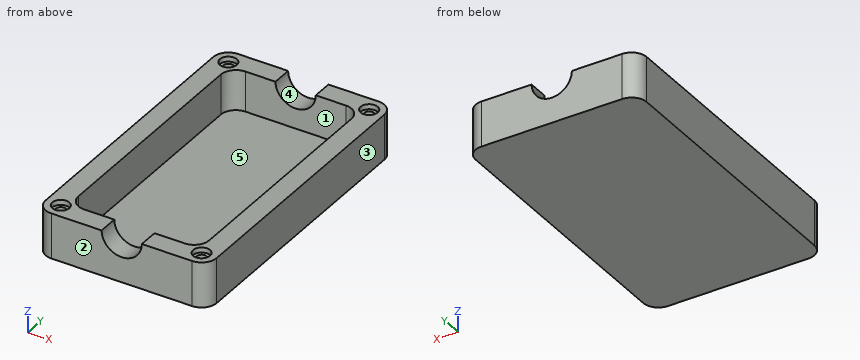
```python
from build123d import *

# Parameters (mm, degrees)
SKETCH008_W                   = 34
SKETCH008_H                   = 59
PAD002_DEPTH                  = 9
SKETCH009_W                   = 26
SKETCH009_H                   = 51
POCKET005_DEPTH               = 8
FILLET003_R                   = 3
SKETCH010_R                   = 1
POCKET006_DEPTH               = 4
SKETCH010_MIRRORED004_2_R     = 1
POCKET006_MIRRORED004_2_DEPTH = 4
SKETCH011_R                   = 1.7
POCKET007_DEPTH               = 1
SKETCH011_MIRRORED006_2_R     = 1.7
POCKET007_MIRRORED006_2_DEPTH = 1
SKETCH016_R                   = 4
POCKET011_DEPTH               = 59.001


with BuildPart() as part:
    # Sketch008 → Pad002 (new body)
    with BuildSketch(Plane.XY):
        Rectangle(SKETCH008_W, SKETCH008_H)
    extrude(amount=PAD002_DEPTH)

    # Sketch009 (on Face6 of Pad002) → Pocket005 (cut)
    with BuildSketch(Plane.XY.offset(9)):
        Rectangle(SKETCH009_W, SKETCH009_H)
    extrude(amount=-POCKET005_DEPTH, mode=Mode.SUBTRACT)

    # Fillet003
    fillet003_edges = [part.edges().sort_by_distance(p)[0] for p in [
        (-13, 25.5, 5),
        (-17, 29.5, 4.5),
        (17, 29.5, 4.5),
        (13, 25.5, 5),
        (17, -29.5, 4.5),
        (13, -25.5, 5),
        (-13, -25.5, 5),
        (-17, -29.5, 4.5),
    ]]
    fillet(fillet003_edges, radius=FILLET003_R)

    # Sketch010 (on Face5 of Fillet003) → Pocket006 (cut)
    with BuildSketch(Plane.XY.offset(9)):
        with Locations((-14, 26.5)):
            Circle(SKETCH010_R)
    pocket006 = extrude(amount=-POCKET006_DEPTH, mode=Mode.SUBTRACT)

    # Sketch010 Mirrored004 2 → Pocket006 Mirrored004 2 (cut)
    with BuildSketch(Plane(origin=(0, 0, 9), x_dir=(-1, 0, 0), z_dir=(0, 0, -1))):
        with Locations((-14, 26.5)):
            Circle(SKETCH010_MIRRORED004_2_R)
    pocket006_mirrored004_2 = extrude(amount=POCKET006_MIRRORED004_2_DEPTH, mode=Mode.SUBTRACT)

    # Mirrored005: Pocket006, Pocket006 Mirrored004 2 across Sketch010 H_Axis
    add(pocket006.mirror(Plane(origin=(0, 0, 9), x_dir=(0, 0, 1), z_dir=(0, 1, 0))), mode=Mode.SUBTRACT)
    add(pocket006_mirrored004_2.mirror(Plane(origin=(0, 0, 9), x_dir=(0, 0, 1), z_dir=(0, 1, 0))), mode=Mode.SUBTRACT)

    # Sketch011 (on Face5 of MultiTransform002) → Pocket007 (cut)
    with BuildSketch(Plane.XY.offset(9)):
        with Locations((-14, 26.5)):
            Circle(SKETCH011_R)
    pocket007 = extrude(amount=-POCKET007_DEPTH, mode=Mode.SUBTRACT)

    # Sketch011 Mirrored006 2 → Pocket007 Mirrored006 2 (cut)
    with BuildSketch(Plane(origin=(0, 0, 9), x_dir=(-1, 0, 0), z_dir=(0, 0, -1))):
        with Locations((-14, 26.5)):
            Circle(SKETCH011_MIRRORED006_2_R)
    pocket007_mirrored006_2 = extrude(amount=POCKET007_MIRRORED006_2_DEPTH, mode=Mode.SUBTRACT)

    # Mirrored007: Pocket007, Pocket007 Mirrored006 2 across Sketch011 H_Axis
    add(pocket007.mirror(Plane(origin=(0, 0, 9), x_dir=(0, 0, 1), z_dir=(0, 1, 0))), mode=Mode.SUBTRACT)
    add(pocket007_mirrored006_2.mirror(Plane(origin=(0, 0, 9), x_dir=(0, 0, 1), z_dir=(0, 1, 0))), mode=Mode.SUBTRACT)

    # Sketch016 (on Face10 of MultiTransform003) → Pocket011 (cut, through all)
    with BuildSketch(Plane.XZ.offset(29.5)):
        with Locations((0, 9)):
            Circle(SKETCH016_R)
    extrude(amount=-POCKET011_DEPTH, mode=Mode.SUBTRACT)


solid = part.part
```
Read the model definition and answer for the solid it produces. Units are mm, in the model's axes. Face numbers are marked on the shaded views. A direction names the side the tool comes from. Give positions to 0.01 mm unless a question says otherwise; leave off trailing zeros. Loops run counter-clockwise (first coordinate to the right, second up) from the corner with the lowest first, then second, coordinate; pieces in that order, holes last.
Item 1: Find the intervals of material crossed by line 1 along Y through (x, z) = (-14, 6.25); line 2 along X through (y, z) = (-12.5, 8.5); line 3 along Z through (x, y) = (10.5, -0.5), in increasing order.
Item 2: The part is cut by section A-A (z = 6.75). Write down the section's boundary in (x, y), and give its area (3 significant figures).
Item 3: For the marked faces 4 and 5, determine the directions among +Z, -Z, +X, -X, +Y, -Y from which every point of the face is accessible in a straight line to the end or side of a thin tool.
Item 4: The part is cut by section B-B (y = -2). Write down the section's boundary in (x, z).
Item 5: The mould has two halves that part along Y. Classify the marked faces 1, 2 and 3: released by +Y, released by -Y, zero draft, split by the parting line, or undercut.
Item 6: The part is cut by section C-C (z = 3.5). Write down the section's boundary in (x, y).
Item 7: The part is cut by section D-D (x = -1.5). Write down the section's boundary in (y, z).
Item 8: Each of these flat-tipped pins is pushed along its axis until it touches: pin 1 Ø1 at (x, y) = (-14.5, -26) entering from +Z; pin 2 Ø6 at (x, y) = (8, -8) entering from +Z; pin 3 Ø1.6 at (x, y) = (14, -26.5) entering from +Z. Where does it stop, or does it pass through?
Taken from the geometry:
1. line 1: y = -29.5 to -27.5, -25.5 to 25.5, 27.5 to 29.5
1. line 2: x = -17 to -13, 13 to 17
1. line 3: z = 0 to 1
2. outline: (-17, -26.5) arc R3 ccw to (-14, -29.5) - (-3.31, -29.5) - (-3.31, -25.5) - (-10, -25.5) arc R3 cw to (-13, -22.5) - (-13, 22.5) arc R3 cw to (-10, 25.5) - (-3.31, 25.5) - (-3.31, 29.5) - (-14, 29.5) arc R3 ccw to (-17, 26.5) - close; (3.31, -29.5) - (14, -29.5) arc R3 ccw to (17, -26.5) - (17, 26.5) arc R3 ccw to (14, 29.5) - (3.31, 29.5) - (3.31, 25.5) - (10, 25.5) arc R3 cw to (13, 22.5) - (13, -22.5) arc R3 cw to (10, -25.5) - (3.31, -25.5) - close; hole circle Ø2 at (-14, -26.5); hole circle Ø2 at (-14, 26.5); hole circle Ø2 at (14, -26.5); hole circle Ø2 at (14, 26.5)
2. area: 615 mm2
3. face 4: +Z, +Y, -Y
3. face 5: +Z
4. outline: (-17, 0) - (17, 0) - (17, 9) - (13, 9) - (13, 1) - (-13, 1) - (-13, 9) - (-17, 9) - close
5. face 1: undercut
5. face 2: released by -Y
5. face 3: zero draft
6. outline: (-17, -26.5) arc R3 ccw to (-14, -29.5) - (14, -29.5) arc R3 ccw to (17, -26.5) - (17, 26.5) arc R3 ccw to (14, 29.5) - (-14, 29.5) arc R3 ccw to (-17, 26.5) - close; hole (-13, -22.5) arc R3 ccw to (-10, -25.5) - (10, -25.5) arc R3 ccw to (13, -22.5) - (13, 22.5) arc R3 ccw to (10, 25.5) - (-10, 25.5) arc R3 ccw to (-13, 22.5) - close
7. outline: (-29.5, 0) - (29.5, 0) - (29.5, 5.29) - (25.5, 5.29) - (25.5, 1) - (-25.5, 1) - (-25.5, 5.29) - (-29.5, 5.29) - close
8. pin 1: stops at z = 8
8. pin 2: stops at z = 1
8. pin 3: stops at z = 5
